from build123d import *

# Parameters (mm, degrees)
SKETCH1_R          = 20
BASE_FLANGE1_DEPTH = 3


# Sheet-metal steps are written as plain solids
with BuildPart() as part:
    # Sketch1 → Base-Flange1 (new body)
    with BuildSketch(Plane(origin=(0, 0, 0), x_dir=(1, 0, 0), z_dir=(0, 1, 0))):
        with BuildLine():
            Line((0, 0), (150, 0))
            ThreePointArc((150, 0), (282.915026221, 60), (150, 120))
            Line((150, 120), (0, 120))
            Line((0, 120), (0, 0))
        make_face()
        with Locations(Location((202.915026221, 60, 0), (0, 0, 270))):
            Circle(SKETCH1_R, mode=Mode.SUBTRACT)
    extrude(amount=-BASE_FLANGE1_DEPTH)


solid = part.part
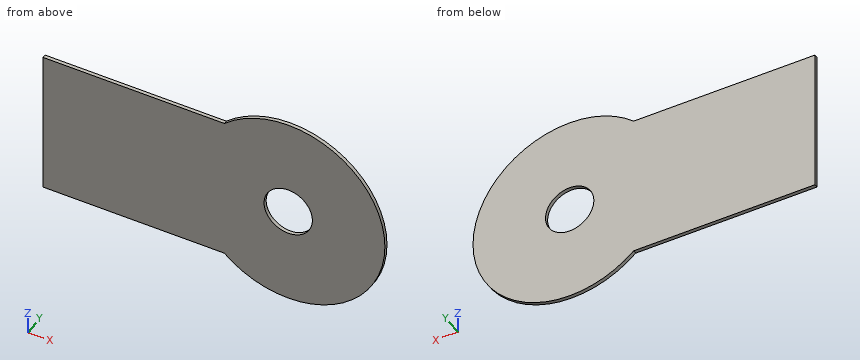
The listing builds one solid part. Answer for the finished solid, in the listing's coordinates (mm). Coordinates: 2 decimals unless noted, no trailing zeros. Write each loop counter-clockwise with the first axis right and the second up, starting at its lowest first coordinate (ties: lowest second). Pieces come first, ordered by that corner, then holes. Notation, with made-up numbers: M 47,-37.5 L 101,-37.5 A32 ccw 101,-3.5 Z; hole C 16,4 d5. An arc over 180 degrees is marked long. Put each result on its own line as item: value. Start each with the question number.
1. A cutting plane is placed at B-B on y = -1.4. Write down the section's boundary in (x, z), then the cut area to 3 significant figures.
2. Flat-ended cylindrical pins translate along their axes: P1, Ø1, axis at x = 127, y = -2.5, coming from the -Z side; P2, Ø0.9, axis at x = 78, y = -1, coming from the +Z side; P3, Ø1, axis at y = -0.5, z = -45.5, coming from the +X side. Find the tip coordinate at first contact, or state that the pin passes through.
3. A cutting plane is placed at A-A on z = -60. Write down the section's boundary in (x, y), then the cut area to 3 significant figures.
4. A cutting plane is placed at C-C on x = 67.5. Write down the section's boundary in (y, z), then the cut area to 3 significant figures.
5. A cutting plane is placed at D-D on z = -105. Write down the section's boundary in (x, y), then the cut area to 3 significant figures.
6. Consider line 1 (X direction, y = -1.9, z = -60); line 2 (Z direction, x = 128, y = -1.65); line 3 (X direction, y = -1.55, z = -63.5). Determine where each line is inside the solid, lowest interval first. Write a range as from..to.
Resolved:
1. outline: M 0,-120 L 150,-120 A80 ccw long 150,0 L 0,0 Z; hole C 202.92,-60 d40
1. area: 34,600 mm2
2. P1: stops at z = -120
2. P2: stops at z = 0
2. P3: stops at x = 281.68
3. outline: M 0,-3 L 182.92,-3 L 182.92,0 L 0,0 Z; M 222.92,-3 L 282.92,-3 L 282.92,0 L 222.92,0 Z
3. area: 729 mm2
4. outline: M -3,-120 L 0,-120 L 0,0 L -3,0 Z
4. area: 360 mm2
5. outline: M 0,-3 L 269.06,-3 L 269.06,0 L 0,0 Z
5. area: 807 mm2
6. line 1: x = 0..182.92, 222.92..282.92
6. line 2: z = -120..0
6. line 3: x = 0..183.22, 222.61..282.84
